Build history of the part. All positions in model axes, mm. Face numbers are marked on the shaded views. A direction names the side the tool comes from. Give positions to 0.01 mm unless a question says otherwise; leave off trailing zeros. Loops run counter-clockwise (first coordinate to the right, second up) from the corner with the lowest first, then second, coordinate; pieces in that order, holes last.
1) Band-saw the part on B-B on z = 62. List the corners of the cut face in (x, y).
2) Wall check: line 1 (X direction, y = 17.5, z = 64). Give the ranges that are in metal, low to high.
3) Flat gauge pin, fed straight in: P1, Ø4, axis at y = 60.79, z = 72.06, coming from the -X side. Where does the tip first touch, or does it go through?
4) Band-saw the part on A-A on x = 11. List the corners of the cut face in (y, z), then the cut area to 3 significant figures.
5) Two-plate mould, pull along X, no slides. Class the marked faces 3, 4, 5 and 6: +X half, -X half, draft (parallel to the pull), parting line (faces both ways), or undercut.
6) 3-axis set-ups, long thin cutter, end or side, ignore diameter. For the marked faces 1 and 2: which of +Z, -Z, +X, -X, +Y, -Y reach the whole face in a straight line?
```python
from build123d import *

# Parameters (mm, degrees)
CROQUIS1_W                       = 80
CROQUIS1_H                       = 80
SALIENTE_EXTRUIR1_DEPTH          = 80
VACIADO1_T                       = -0.6
TALADRO_DE_MARGEN_PARA_M41_D     = 4.5
TALADRO_DE_MARGEN_PARA_M41_DEPTH = 5


with BuildPart() as part:
    # Croquis1 → Saliente-Extruir1 (new body)
    with BuildSketch(Plane.XY):
        with Locations((40, 40)):
            Rectangle(CROQUIS1_W, CROQUIS1_H)
    extrude(amount=SALIENTE_EXTRUIR1_DEPTH)

    # Vaciado1
    vaciado1_openings = [part.faces().sort_by_distance(p)[0] for p in [
        (40, 40, 80),
        (40, 40, 0),
    ]]
    offset(amount=VACIADO1_T, openings=vaciado1_openings, kind=Kind.INTERSECTION)

    # Taladro de margen para M41
    with Locations(Plane(origin=(0, -79.637122061, 0), x_dir=(0, 1, 0), z_dir=(-1, 0, 0))):
        with Locations((98.1889532, -72.0625), (140.429406251, -72.0625)):
            Hole(TALADRO_DE_MARGEN_PARA_M41_D / 2, depth=TALADRO_DE_MARGEN_PARA_M41_DEPTH)


solid = part.part
```
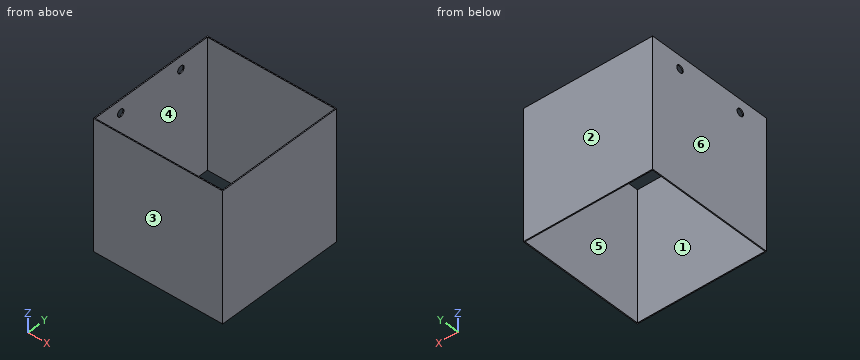
Findings below:
1. outline: (0, 0) - (80, 0) - (80, 80) - (0, 80) - close; hole (0.6, 0.6) - (79.4, 0.6) - (79.4, 79.4) - (0.6, 79.4) - close
2. line 1: x = 0 to 0.6, 79.4 to 80
3. P1: stops at x = 79.4
4. outline: (0, 0) - (0.6, 0) - (0.6, 80) - (0, 80) - close; (79.4, 0) - (80, 0) - (80, 80) - (79.4, 80) - close
4. area: 96.0 mm2
5. face 3: draft
5. face 4: undercut
5. face 5: undercut
5. face 6: -X half
6. face 1: +Z, -Z
6. face 2: +Z, -Z, +X, -X, +Y
